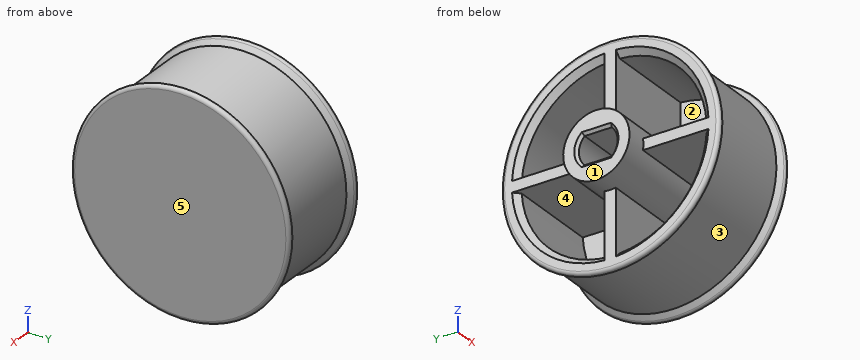
```python
from build123d import *

# Parameters (mm, degrees)
REDONDEO2_R             = 0.5
MOVER_CARA1_BY          = 0.6
CROQUIS3_R              = 4.8
CROQUIS3_R_2            = 2.8
SALIENTE_EXTRUIR1_DEPTH = 17
NERVIO4_REACH           = 28.904
CROQUIS5_WALLS_W        = 1.6
CROQUIS5_WALLS_H        = 65.245471754
MATRIZC1_COUNT          = 4
CHAFL_N1_SIZE           = 0.4


# Read off the part's stored shape, not the designer's step: Vaciado1
with BuildPart() as part:
    # Croquis2 → Revolución1 (revolve)
    with BuildSketch(Plane.XY, mode=Mode.PRIVATE) as revoluci_n1_sk:
        Polygon((-7.5, 0), (7.5, 0), (7.5, 16.5), (6, 15), (-6, 15), (-7.5, 16.5), align=None)
    revolve(revoluci_n1_sk.sketch.rotate(Axis((-7.5, 0, 0), (1, 0, 0)), 90), axis=Axis((-7.5, 0, 0), (1, 0, 0)))

    # Vaciado1 outline → Vaciado1 (revolve, cut)
    with BuildSketch(Plane.YX):
        Polygon((13.4, 5.9), (0, 5.9), (0, -7.5), (14.2372583, -7.5), (13.4, -6.6627417), align=None)
    revolve(axis=Axis((0, 0, 0), (1, 0, 0)), mode=Mode.SUBTRACT)

    # Redondeo2
    redondeo2_edges = [part.edges().sort_by_distance(p)[0] for p in [
        (-7.5, 0, -16.5),
        (7.5, 0, -16.5),
    ]]
    fillet(redondeo2_edges, radius=REDONDEO2_R)

    # Mover cara1: a face moved inward by 0.6
    extrude(part.faces().sort_by_distance((5.9, 0, 0))[0], amount=MOVER_CARA1_BY, dir=(1, 0, 0), mode=Mode.SUBTRACT)

    # Croquis3 → Saliente-Extruir1 (add)
    # profile 1 of 3: a face of its own
    with BuildSketch(Plane.ZY.offset(-6.5)):
        Circle(CROQUIS3_R)
        Circle(CROQUIS3_R_2, mode=Mode.SUBTRACT)
    # profile 2 of 3: a face of its own
    with BuildSketch(Plane.ZY.offset(-6.5)):
        with BuildLine():
            ThreePointArc((2.8, 0), (2.592296279, 1.058300524), (2, 1.959591794))
            Line((2, 1.959591794), (2, -1.959591794))
            ThreePointArc((2, -1.959591794), (2.592296279, -1.058300524), (2.8, 0))
        make_face()
    # profile 3 of 3: a face of its own
    with BuildSketch(Plane.ZY.offset(-6.5)):
        with BuildLine():
            Line((-2, -1.959591794), (-2, 1.959591794))
            ThreePointArc((-2, 1.959591794), (-2.8, 0), (-2, -1.959591794))
        make_face()
    extrude(amount=SALIENTE_EXTRUIR1_DEPTH)

    # Croquis5 walls → Nervio4 (add, up to next)
    with BuildSketch(Plane.ZY.offset(7.5), mode=Mode.PRIVATE) as nervio4_sk1:
        with Locations((0, 9.51862915)):
            Rectangle(CROQUIS5_WALLS_W, CROQUIS5_WALLS_H)
    nervio4_tool1 = extrude(nervio4_sk1.sketch, amount=-NERVIO4_REACH, mode=Mode.PRIVATE) - part.part
    nervio4 = nervio4_tool1.solids().sort_by_distance((-7.5, 9.51862915, 0))[0]
    add(nervio4)

    # MatrizC1: Nervio4 ×4 about axis
    matrizc1_axis = Axis((0, 0, 0), (1, 0, 0))
    for i in range(1, MATRIZC1_COUNT):
        add(nervio4.rotate(matrizc1_axis, i * 360 / MATRIZC1_COUNT))

    # Chaflán1
    chafl_n1_edges = [part.edges().sort_by_distance(p)[0] for p in [
        (-10.5, 0, -2),
        (-10.5, 2.8, 0),
        (-10.5, -2.8, 0),
        (-10.5, 0, 2),
    ]]
    chamfer(chafl_n1_edges, length=CHAFL_N1_SIZE)


solid = part.part
```
Geometry: final body of the model. Coordinates: model frame, mm. Face numbers are marked on the shaded views. A direction names the side the tool comes from. Coordinates: 2 decimals unless noted, no trailing zeros. Order: outer loops, then holes, each group sorted by start corner. A loop starts at its lowest first (then second) coordinate and runs counter-clockwise, first axis right, second up.
Item 1: Contact query for flat-ended pins moving along their axis: P1, Ø2, axis at x = -1.5, z = 3.5, coming from the -Y side; P2, Ø1, axis at x = -2.5, y = -5.5, coming from the -Z side; P3, Ø10, axis at x = -3.5, z = 5.5, coming from the +Y side. Output: stop coordinate, or through.
Answer:
P1: stops at y = -14.79
P2: stops at z = -14.14
P3: stops at y = 15.68
Item 2: Section query A-A (x = -0.5). Output: boundary loops of the cut face in (y, z).
Answer:
outline: circle Ø30 at (0, 0); hole (-13.38, -0.8) arc R13.4 ccw to (-0.8, -13.38) - (-0.8, -4.73) arc R4.8 cw to (-4.73, -0.8) - close; hole (-13.38, 0.8) - (-4.73, 0.8) arc R4.8 cw to (-0.8, 4.73) - (-0.8, 13.38) arc R13.4 ccw to start; hole (-1.96, -2) - (1.96, -2) arc R2.8 ccw to (1.96, 2) - (-1.96, 2) arc R2.8 ccw to start; hole (0.8, -13.38) arc R13.4 ccw to (13.38, -0.8) - (4.73, -0.8) arc R4.8 cw to (0.8, -4.73) - close; hole (0.8, 4.73) arc R4.8 cw to (4.73, 0.8) - (13.38, 0.8) arc R13.4 ccw to (0.8, 13.38) - close
Item 3: Access query for the marked faces 1 and 2. Directions: +Z, -Z, +X, -X, +Y, -Y. A direction counts if a zero-diameter tool reaches every point of the face in a straight line with its end or side. Return the directions, or none.
Answer:
face 1: +Z, -Z, -X, +Y, -Y
face 2: -X
Item 4: Draft query along Z for the marked faces 3, 4 and 5. Return one class per face: released by +Z, released by -Z, zero draft, split by the parting line, or undercut.
Answer:
face 3: split by the parting line
face 4: undercut
face 5: zero draft
Item 5: Material intervals for line 1 along Y through (x, z) = (-7, 11.5); line 2 along Z through (x, y) = (-2, -11); line 3 along Z through (x, y) = (-2.5, -9.5), sorted ascending.
Answer:
line 1: y = -10.82 to -7.51, -0.8 to 0.8, 7.51 to 10.82
line 2: z = -10.2 to -7.65, -0.8 to 0.8, 7.65 to 10.2
line 3: z = -11.61 to -9.45, -0.8 to 0.8, 9.45 to 11.61
Item 6: Section query C-C (z = 0). Output: boundary loops of the cut face in (x, y), then the cut area to 3 significant figures.
Answer:
outline: (-10.5, -4.8) - (-7.5, -4.8) - (-7.5, -15.29) arc R0.5 ccw to (-6.65, -15.65) - (-6, -15) - (6, -15) - (6.65, -15.65) arc R0.5 ccw to (7.5, -15.29) - (7.5, 15.29) arc R0.5 ccw to (6.65, 15.65) - (6, 15) - (-6, 15) - (-6.65, 15.65) arc R0.5 ccw to (-7.5, 15.29) - (-7.5, 4.8) - (-10.5, 4.8) - (-10.5, 3.2) - (-10.1, 2.8) - (6.5, 2.8) - (6.5, -2.8) - (-10.1, -2.8) - (-10.5, -3.2) - close
area: 387 mm2
Item 7: Section query B-B (y = 0). Output: boundary loops of the cut face in (x, z).
Answer:
outline: (-10.5, -4.8) - (-7.5, -4.8) - (-7.5, -15.29) arc R0.5 ccw to (-6.65, -15.65) - (-6, -15) - (6, -15) - (6.65, -15.65) arc R0.5 ccw to (7.5, -15.29) - (7.5, 15.29) arc R0.5 ccw to (6.65, 15.65) - (6, 15) - (-6, 15) - (-6.65, 15.65) arc R0.5 ccw to (-7.5, 15.29) - (-7.5, 4.8) - (-10.5, 4.8) - (-10.5, 2.4) - (-10.1, 2) - (6.5, 2) - (6.5, -2) - (-10.1, -2) - (-10.5, -2.4) - close
